Geometry: final body of the model. Coordinates: model frame, mm. A direction names the side the tool comes from. Give positions to 0.01 mm unless a question says otherwise; leave off trailing zeros. Order: outer loops, then holes, each group sorted by start corner. A loop starts at its lowest first (then second) coordinate and runs counter-clockwise, first axis right, second up. Notation, with made-up numbers: (34, 29.5) - (77, 29.5) arc R25 cw to (77, 43.5) - close; hole circle Ø10 at (18.5, -34.75). An arc over 180 degrees is marked (long way). Put each result on its own line as item: value. Start each with the question number.
1. Section D-D on y = -6. Return the cut outline in (x, z), plus the area to 3 significant figures.
2. Ray query, line 1 along Z through (x, y) = (5, 24.5); line 2 along Z through (x, y) = (7, 13); line 3 along X through (y, z) = (-18.5, 14.5). Return the intervals inside material, ascending. Write a range as from..to.
3. Mould query, pull axis X, two halves, no side actions, for faces 1 (the cylindrical face through (-8.676, 1.563, 92.811)), 2 (the cylindrical face through (-21.86, -24.31, 37.01)), 3 (the flat face through (-5, 3, 0)), 4 (the cylindrical face through (-30.204, -19.046, 75.535)). Classes: pulls with the +X half, pulls with the -X half, needs draft (parallel to the pull), parting line crosses it, or undercut.
4. Section B-B on y = -22. Return the cut outline in (x, z), plus the area to 3 significant figures.
5. First-contact query: P1, Ø2, axis at x = 17.5, z = 15, coming from the -Y side; P2, Ø16.5, axis at x = -24, y = -17.5, coming from the -Z side; P3, Ø8, axis at x = 18.64, y = 26.26, coming from the +Z side; P4, Ø6, axis at x = 18.64, y = -20.74, coming from the -Z side. Flat tips, straight axial feed; report the tip coordinate or a pass-through.
6. Set-up query: faces 5 (the cylindrical face through (-20, -8.8, 78.7)), 6 (the cylindrical face through (-21.858, 29.838, 37.011)), 7 (the cylindrical face through (22.213, -14.232, 37.011)). Return all of +Z, -Z, +X, -X, +Y, -Y with unobstructed straight access to the full face (end or side cutting, diameter ignored); none if empty.
7. Section C-C on x = -14.5. Return the cut outline in (y, z).
from build123d import *

# Parameters (mm, degrees)
SKETCH1_W            = 57
SKETCH1_H            = 57
BOSS_EXTRUDE1_DEPTH  = 78
SKETCH2_W            = 10
SKETCH2_H            = 10
CUT_EXTRUDE1_DEPTH   = 73
LPATTERN1_COUNT      = 2
LPATTERN1_PITCH      = 47
LPATTERN1_COUNT_DIR2 = 2
LPATTERN1_PITCH_DIR2 = 47
SKETCH3_R            = 2.5
CUT_EXTRUDE2_DEPTH   = 50
LPATTERN2_COUNT      = 2
LPATTERN2_PITCH      = 47
LPATTERN2_COUNT_DIR2 = 2
LPATTERN2_PITCH_DIR2 = 47
FILLET1_R            = 5
SKETCH5_R            = 19.05
BOSS_EXTRUDE3_DEPTH  = 1.5
SKETCH4_R            = 4
BOSS_EXTRUDE2_DEPTH  = 28.5


with BuildPart() as part:
    # Sketch1 → Boss-Extrude1 (new body)
    with BuildSketch(Plane.XY):
        with Locations((-4.861204013, 2.764214047)):
            Rectangle(SKETCH1_W, SKETCH1_H)
    extrude(amount=BOSS_EXTRUDE1_DEPTH)

    # Sketch2 → Cut-Extrude1 (cut)
    with BuildSketch(Plane(origin=(0, 0, 0), x_dir=(-1, 0, 0), z_dir=(0, 0, -1))):
        with Locations((-18.638795987, 26.264214047)):
            Rectangle(SKETCH2_W, SKETCH2_H)
    cut_extrude1 = extrude(amount=-CUT_EXTRUDE1_DEPTH, mode=Mode.SUBTRACT)

    # LPattern1: Cut-Extrude1 2 × 2
    with Locations(*[(-i * LPATTERN1_PITCH, -j * LPATTERN1_PITCH_DIR2, 0) for i in range(LPATTERN1_COUNT) for j in range(LPATTERN1_COUNT_DIR2) if (i, j) != (0, 0)]):
        add(cut_extrude1, mode=Mode.SUBTRACT)

    # Sketch3 → Cut-Extrude2 (cut)
    with BuildSketch(Plane.XY.offset(78)):
        with Locations((-28.361204013, 26.264214047)):
            Circle(SKETCH3_R)
    cut_extrude2 = extrude(amount=-CUT_EXTRUDE2_DEPTH, mode=Mode.SUBTRACT)

    # LPattern2: Cut-Extrude2 2 × 2
    with Locations(*[(i * LPATTERN2_PITCH, -j * LPATTERN2_PITCH_DIR2, 0) for i in range(LPATTERN2_COUNT) for j in range(LPATTERN2_COUNT_DIR2) if (i, j) != (0, 0)]):
        add(cut_extrude2, mode=Mode.SUBTRACT)

    # Fillet1
    fillet1_edges = [part.edges().sort_by_distance(p)[0] for p in [
        (-33.361204013, 21.264214047, 36.5),
        (-23.361204013, 21.264214047, 36.5),
        (-23.361204013, 31.264214047, 36.5),
        (13.638795987, 31.264214047, 36.5),
        (13.638795987, 21.264214047, 36.5),
        (23.638795987, 21.264214047, 36.5),
        (23.638795987, -25.735785953, 75.5),
        (23.638795987, -15.735785953, 36.5),
        (13.638795987, -15.735785953, 36.5),
        (13.638795987, -25.735785953, 36.5),
        (-23.361204013, -25.735785953, 36.5),
        (-23.361204013, -15.735785953, 36.5),
        (-33.361204013, -15.735785953, 36.5),
        (-33.361204013, -25.735785953, 75.5),
        (-33.361204013, 31.264214047, 75.5),
        (23.638795987, 31.264214047, 75.5),
    ]]
    fillet(fillet1_edges, radius=FILLET1_R - 0.0001)  # a hair under: the kernel refuses the full size

    # Sketch5 → Boss-Extrude3 (add)
    with BuildSketch(Plane.XY.offset(78)):
        with Locations((-4.861204013, 2.764214047)):
            Circle(SKETCH5_R)
    extrude(amount=BOSS_EXTRUDE3_DEPTH)

    # Sketch4 → Boss-Extrude2 (add)
    with BuildSketch(Plane.XY.offset(78)):
        with Locations(Location((-4.861204013, 2.764214047, 0), (0, 0, 180))):
            Circle(SKETCH4_R)
    extrude(amount=BOSS_EXTRUDE2_DEPTH)


solid = part.part
Resolved:
1. outline: (-33.36, 0) - (23.64, 0) - (23.64, 78) - (12.05, 78) - (12.05, 79.5) - (-21.78, 79.5) - (-21.78, 78) - (-33.36, 78) - close
1. area: 4,500 mm^2
2. line 1: 0..78
2. line 2: 0..79.5
2. line 3: -23.89..14.17
3. face 1: parting line crosses it
3. face 2: pulls with the -X half
3. face 3: needs draft
3. face 4: undercut
4. outline: (-33.2, 73) - (-30.52, 73) - (-30.52, 78) - (-33.2, 78) - close; (-26.2, 73) - (-23.2, 73) - (-23.2, 0) - (13.48, 0) - (13.48, 73) - (16.48, 73) - (16.48, 78) - (-26.2, 78) - close; (20.8, 73) - (23.48, 73) - (23.48, 78) - (20.8, 78) - close
4. area: 2,920 mm^2
5. P1: y = -16.22
5. P2: z = 0
5. P3: z = 78
5. P4: z = 73
6. face 5: +Z
6. face 6: -Z, -X, +Y
6. face 7: -Z, +X, -Y
7. outline: (-25.74, 0) - (31.26, 0) - (31.26, 78) - (19.2, 78) - (19.2, 79.5) - (-13.67, 79.5) - (-13.67, 78) - (-25.74, 78) - close
